from build123d import *

# Parameters (mm, degrees)
SKETCH4_R                 = 42.545
BOSS_EXTRUDE2_DEPTH       = 5.207
SKETCH5_R                 = 29.845
CUT_EXTRUDE5_DEPTH        = 6.207
CUT_EXTRUDE11_DEPTH       = 6.207
F_6_32_TAPPED_HOLE1_D     = 2.7051
F_2_56_TAPPED_HOLE1_D     = 1.778
F_2_56_TAPPED_HOLE1_DEPTH = 3.302
F_2_56_TAPPED_HOLE1_TIP   = 0.53416509


with BuildPart() as part:
    # Sketch4 → Boss-Extrude2 (new body)
    with BuildSketch(Plane.XY):
        Circle(SKETCH4_R)
    extrude(amount=BOSS_EXTRUDE2_DEPTH)

    # Sketch5 → Cut-Extrude5 (cut, through all)
    with BuildSketch(Plane.XY.offset(5.207)):
        Circle(SKETCH5_R)
    extrude(amount=-CUT_EXTRUDE5_DEPTH, mode=Mode.SUBTRACT)

    # Sketch8 → Cut-Extrude11 (cut, through all)
    with BuildSketch(Plane.XY.offset(5.207)):
        Polygon((45.273745286, 20.127637411), (26.500513186, 12.351510066), (27.472529104, 10.004856053), (46.245761204, 17.780983399), align=None)
        Polygon((17.697597616, 39.407110255), (15.350943603, 40.379126173), (14.864935644, 39.205799167), (17.211589657, 38.233783248), align=None)
        Polygon((-15.350943603, 40.379126173), (-17.697597616, 39.407110255), (-17.211589657, 38.233783248), (-14.864935644, 39.205799167), align=None)
        Polygon((-39.407110255, 17.697597616), (-40.379126173, 15.350943603), (-39.205799167, 14.864935644), (-38.233783248, 17.211589657), align=None)
        Polygon((-40.379126173, -15.350943603), (-39.407110255, -17.697597616), (-38.233783248, -17.211589657), (-39.205799167, -14.864935644), align=None)
        Polygon((-17.697597616, -39.407110255), (-15.350943603, -40.379126173), (-14.864935644, -39.205799167), (-17.211589657, -38.233783248), align=None)
        Polygon((15.350943603, -40.379126173), (17.697597616, -39.407110255), (17.211589657, -38.233783248), (14.864935644, -39.205799167), align=None)
        Polygon((39.407110255, -17.697597616), (40.379126173, -15.350943603), (39.205799167, -14.864935644), (38.233783248, -17.211589657), align=None)
    extrude(amount=-CUT_EXTRUDE11_DEPTH, mode=Mode.SUBTRACT)

    # #6-32 Tapped Hole1 (through all)
    with Locations(Plane.XY.offset(5.207)):
        with Locations((36.195, 0), (25.593729945, -25.593729945), (0, -36.195), (-25.593729945, -25.593729945), (-36.195, 0), (-25.593729945, 25.593729945), (0, 36.195), (25.593729945, 25.593729945)):
            Hole(F_6_32_TAPPED_HOLE1_D / 2)

    # #2-56 Tapped Hole1
    with Locations(Plane.XY.offset(5.207)):
        with Locations((13.851226834, 33.439819679), (-13.851226834, 33.439819679), (-33.439819679, 13.851226834), (-33.439819679, -13.851226834), (-13.851226834, -33.439819679), (13.851226834, -33.439819679), (33.439819679, -13.851226834), (33.439819679, 13.851226834)):
            Hole(F_2_56_TAPPED_HOLE1_D / 2, depth=F_2_56_TAPPED_HOLE1_DEPTH)
            with Locations((0, 0, -(F_2_56_TAPPED_HOLE1_DEPTH + F_2_56_TAPPED_HOLE1_TIP / 2))):  # 118° drill point
                Cone(0, F_2_56_TAPPED_HOLE1_D / 2, F_2_56_TAPPED_HOLE1_TIP, mode=Mode.SUBTRACT)


solid = part.part
Geometry: final body of the model. Coordinates: model frame, mm. A direction names the side the tool comes from. Give positions to 0.01 mm unless a question says otherwise; leave off trailing zeros. Write each loop counter-clockwise with the first axis right and the second up, starting at its lowest first coordinate (ties: lowest second). Pieces come first, ordered by that corner, then holes. Notation, with made-up numbers: (36, 68.25) -> (88, 68.25) arc R11 ccw to (88, 82.25) -> close; hole circle Ø3 at (32, -4). An arc over 180 degrees is marked (long way). Answer as a JSON object with one key per item and string values.
1. Cut plane C-C on x = -20. Output: boundary loops of the cut face in (y, z).
Ans:
{"outline": "(-37.55, 0) -> (-22.15, 0) -> (-22.15, 5.21) -> (-37.55, 5.21) -> close; (22.15, 0) -> (37.55, 0) -> (37.55, 5.21) -> (22.15, 5.21) -> close"}
2. Contact query for flat-ended pins moving along their axis: pin 1 (4.5 mm diameter, centred on x = 36.195, y = 0, fed in from +Z); pin 2 (3 mm diameter, centred on x = 18, z = 3, fed in from +Y); pin 3 (2 mm diameter, centred on x = 8, z = 4.5, fed in from +Y); pin 4 (1.4 mm diameter, centred on x = -33.44, y = -13.85, fed in from +Z). Output: stop coordinate, or through.
Ans:
{"pin 1": "stops at z = 5.21", "pin 2": "stops at y = 38.8", "pin 3": "stops at y = 41.97", "pin 4": "stops at z = 1.79"}
3. Ray query, probe 1 along Y at (x, z) = (0, 2.3) (3 decimals); probe 2 along X at (y, z) = (13.5, 2.8); probe 3 along X at (y, z) = (26.5, 1.95). Return the intervals inside material, ascending. Write a range as from..to.
Ans:
{"probe 1": "y = -42.545..-37.548, -34.842..-29.845, 29.845..34.842, 37.548..42.545", "probe 2": "x = -40.35..-34.26, -32.62..-26.62, 26.62..29.27, 35.91..40.35", "probe 3": "x = -33.28..-26.6, -24.59..-13.73, 13.73..24.59, 26.6..33.28"}
4. Mould query, pull axis Y, two halves, no side actions, for faces 3 (the flat face through (-10, 29, 5.207)), 4 (the cylindrical face through (24.867, 26.734, 2.567)), 5 (the cylindrical face through (42.544, -0.216, 2.567)). Classes: pulls with the +Y half, pulls with the -Y half, needs draft (parallel to the pull), parting line crosses it, or undercut.
Ans:
{"face 3": "needs draft", "face 4": "undercut", "face 5": "parting line crosses it"}
5. Access query for faces 1 (the cylindrical face through (-0.216, -42.544, 2.567)), 2 (the flat face through (33.015, 15.05, 2.64)). Directions: +Z, -Z, +X, -X, +Y, -Y. A direction counts if a zero-diameter tool reaches every point of the face in a straight line with its end or side. Return the directions, or none.
Ans:
{"face 1": "+Z, -Z, -Y", "face 2": "+Z, -Z"}
6. Cut plane A-A on y = 0. Output: boundary loops of the cut face in (x, z) (3 decimals).
Ans:
{"outline": "(-42.545, 0) -> (-37.548, 0) -> (-37.548, 5.207) -> (-42.545, 5.207) -> close; (-34.842, 0) -> (-29.845, 0) -> (-29.845, 5.207) -> (-34.842, 5.207) -> close; (29.845, 0) -> (34.842, 0) -> (34.842, 5.207) -> (29.845, 5.207) -> close; (37.548, 0) -> (42.545, 0) -> (42.545, 5.207) -> (37.548, 5.207) -> close"}
7. Cut plane D-D on y = 20.5. Output: boundary loops of the cut face in (x, z), and give its area (3 significant figures).
Ans:
{"outline": "(-37.28, 0) -> (-21.69, 0) -> (-21.69, 5.21) -> (-37.28, 5.21) -> close; (21.69, 0) -> (37.28, 0) -> (37.28, 5.21) -> (21.69, 5.21) -> close", "area": "162 mm^2"}
